Answer from the drawing. Dimensions are ordinates in mm from the lowest x, y and z of the part. A direction names the side the tool comes from. Round coordinates to 2 decimals unless told otherwise and drop trailing zeros. Loops run counter-clockwise (first coordinate to the right, second up) from the corner with the lowest first, then second, coordinate; pieces in that order, holes last. Notation, with made-up numbers: M -17,-28 L 18,-28 A21 ccw 18,-14 Z; hole C 10,-17 d1. An arc over 180 degrees is marked long. One line per item, written item: value.
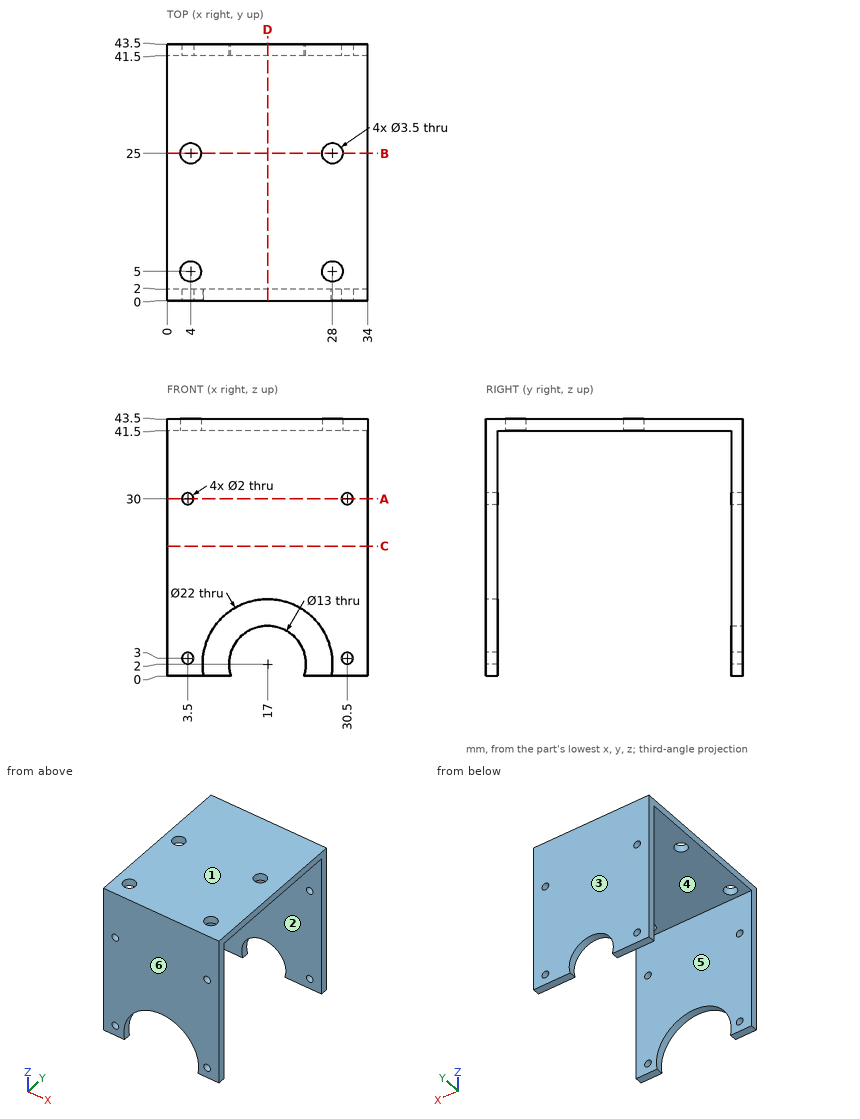
1) Find section C-C (z = 22). Give the vertices of the cut face in (x, y).
Check values:
outline: M 0,0 L 34,0 L 34,2 L 0,2 Z; M 0,41.5 L 34,41.5 L 34,43.5 L 0,43.5 Z
2) This flat-tipped pin is pushed along its axis until it touches: pin 1 (10 mm diameter, centred on x = 11.5, y = 25.5, fed in from -Z). Where does it stop, or does it pass through?
Check values:
pin 1: z = 41.5
3) Find section A-A (z = 30). Give the vertices of the cut face in (x, y), then the cut area to 3 significant figures.
Check values:
outline: M 0,0 L 2.5,0 L 2.5,2 L 0,2 Z; M 0,41.5 L 2.5,41.5 L 2.5,43.5 L 0,43.5 Z; M 4.5,0 L 29.5,0 L 29.5,2 L 4.5,2 Z; M 4.5,41.5 L 29.5,41.5 L 29.5,43.5 L 4.5,43.5 Z; M 31.5,0 L 34,0 L 34,2 L 31.5,2 Z; M 31.5,41.5 L 34,41.5 L 34,43.5 L 31.5,43.5 Z
area: 120 mm2
4) Find the intervals of material crossed by probe 1 along Z at (x, y) = (3.5, 0.95); probe 2 along X at (y, z) = (1, 30); probe 3 along Y at (x, z) = (28, 42.45), in increasing order. Write a range as from..to.
Check values:
probe 1: 0..2, 4..29, 31..43.5
probe 2: 0..2.5, 4.5..29.5, 31.5..34
probe 3: 0..3.25, 6.75..23.25, 26.75..43.5
5) Find section B-B (y = 25). Give the vertices of the cut face in (x, z), then the cut area to 3 significant figures.
Check values:
outline: M 0,41.5 L 2.25,41.5 L 2.25,43.5 L 0,43.5 Z; M 5.75,41.5 L 26.25,41.5 L 26.25,43.5 L 5.75,43.5 Z; M 29.75,41.5 L 34,41.5 L 34,43.5 L 29.75,43.5 Z
area: 54.0 mm2
6) For the marked faces 1 and 2, determine the directions among +Z, -Z, +X, -X, +Y, -Y from which every point of the face is accessible in a straight line to the end or side of a thin tool.
Check values:
face 1: +Z, +X, -X, +Y, -Y
face 2: -Z, +X, -X
7) The mould has two halves that part along Y. Classify the marked faces 3, 4, 5 and 6: +Y half, -Y half, draft (parallel to the pull), parting line (faces both ways), or undercut.
Check values:
face 3: +Y half
face 4: undercut
face 5: undercut
face 6: -Y half
8) Find section D-D (x = 17). Give the vertices of the cut face in (y, z), then the cut area to 3 significant figures.
Check values:
outline: M 0,13 L 2,13 L 2,41.5 L 41.5,41.5 L 41.5,8.5 L 43.5,8.5 L 43.5,43.5 L 0,43.5 Z
area: 210 mm2
